Work out the finished part from the listing and answer in its coordinate system (mm). Give positions to 0.01 mm unless a question says otherwise; leave off trailing zeros. Loops run counter-clockwise (first coordinate to the right, second up) from the corner with the lowest first, then second, coordinate; pieces in that order, holes last. Notation, with made-up numbers: M -23,3 L 12,3 A23 ccw 12,29 Z; hole C -3.75,84 d10. An arc over 180 degrees is marked long. Answer in a Markdown table with one row per item. Add a question column.
from build123d import *

# Parameters (mm, degrees)
SKETCH1_R             = 92.075
BOSS_EXTRUDE1_DEPTH   = 4.7625
FILLET1_R             = 6.35
SKETCH4_R             = 1.5875
CUT_EXTRUDE1_DEPTH    = 131.30077765
SKETCH5_R             = 2.38125
CUT_EXTRUDE2_DEPTH    = 131.30077765
FRONTPATERNCOPY_COUNT = 18


with BuildPart() as part:
    # Sketch1 → Boss-Extrude1 (new body)
    with BuildSketch(Plane.XY):
        with Locations(Location((0, 0, 0), (0, 0, 180))):
            Circle(SKETCH1_R)
        with BuildLine():
            Line((-45.8597, 4.659861673), (-45.8597, 11.409392412))
            Line((-45.8597, 11.409392412), (-51.623596361, 20.547401417))
            ThreePointArc((-51.623596361, 20.547401417), (-49.007713262, 26.180822124), (-45.779418198, 31.487081093))
            Line((-45.779418198, 31.487081093), (-35.046071586, 32.720361416))
            Line((-35.046071586, 32.720361416), (-29.200806502, 36.095126785))
            ThreePointArc((-29.200806502, 36.095126785), (-27.113011458, 44.379898214), (-18.894291413, 42.045596046))
            Line((-18.894291413, 42.045596046), (-13.04902633, 45.420361416))
            Line((-13.04902633, 45.420361416), (-8.017226572, 54.981046592))
            ThreePointArc((-8.017226572, 54.981046592), (-1.830599579, 55.532335728), (4.378903018, 55.389679676))
            Line((4.378903018, 55.389679676), (10.813628414, 46.710969004))
            Line((10.813628414, 46.710969004), (16.658893498, 43.336203635))
            ThreePointArc((16.658893498, 43.336203635), (24.877613542, 45.670505803), (26.965408587, 37.385734374))
            Line((26.965408587, 37.385734374), (32.81067367, 34.010969004))
            Line((32.81067367, 34.010969004), (43.606369789, 34.433645175))
            ThreePointArc((43.606369789, 34.433645175), (47.177113682, 29.351513604), (50.158321216, 23.902598583))
            Line((50.158321216, 23.902598583), (45.8597, 13.990607588))
            Line((45.8597, 13.990607588), (45.8597, 7.241076849))
            ThreePointArc((45.8597, 7.241076849), (51.990625, 1.290607588), (45.8597, -4.659861673))
            Line((45.8597, -4.659861673), (45.8597, -11.409392412))
            Line((45.8597, -11.409392412), (51.623596361, -20.547401417))
            ThreePointArc((51.623596361, -20.547401417), (49.007713262, -26.180822124), (45.779418198, -31.487081093))
            Line((45.779418198, -31.487081093), (35.046071586, -32.720361416))
            Line((35.046071586, -32.720361416), (29.200806502, -36.095126785))
            ThreePointArc((29.200806502, -36.095126785), (27.113011458, -44.379898214), (18.894291413, -42.045596046))
            Line((18.894291413, -42.045596046), (13.04902633, -45.420361416))
            Line((13.04902633, -45.420361416), (8.017226572, -54.981046592))
            ThreePointArc((8.017226572, -54.981046592), (1.830599579, -55.532335728), (-4.378903018, -55.389679676))
            Line((-4.378903018, -55.389679676), (-10.813628414, -46.710969004))
            Line((-10.813628414, -46.710969004), (-16.658893498, -43.336203635))
            ThreePointArc((-16.658893498, -43.336203635), (-24.877613542, -45.670505803), (-26.965408587, -37.385734374))
            Line((-26.965408587, -37.385734374), (-32.81067367, -34.010969004))
            Line((-32.81067367, -34.010969004), (-43.606369789, -34.433645175))
            ThreePointArc((-43.606369789, -34.433645175), (-47.177113682, -29.351513604), (-50.158321216, -23.902598583))
            Line((-50.158321216, -23.902598583), (-45.8597, -13.990607588))
            Line((-45.8597, -13.990607588), (-45.8597, -7.241076849))
            ThreePointArc((-45.8597, -7.241076849), (-51.990625, -1.290607588), (-45.8597, 4.659861673))
        make_face(mode=Mode.SUBTRACT)
    extrude(amount=BOSS_EXTRUDE1_DEPTH)

    # Fillet1
    fillet1_edges = [part.edges().sort_by_distance(p)[0] for p in [
        (-43.606369789, -34.433645175, 2.38125),
        (-4.378903018, -55.389679676, 2.38125),
        (8.017226572, -54.981046592, 2.38125),
        (45.779418198, -31.487081093, 2.38125),
        (51.623596361, -20.547401417, 2.38125),
        (50.158321216, 23.902598583, 2.38125),
        (43.606369789, 34.433645175, 2.38125),
        (4.378903018, 55.389679676, 2.38125),
        (-8.017226572, 54.981046592, 2.38125),
        (-45.779418198, 31.487081093, 2.38125),
        (-51.623596361, 20.547401417, 2.38125),
        (-50.158321216, -23.902598583, 2.38125),
    ]]
    fillet(fillet1_edges, radius=FILLET1_R)

    # Sketch4 → Cut-Extrude1 (cut, through all)
    with BuildSketch(Plane.XY.offset(4.7625)):
        with Locations((-16.953011458, 50.011322779)):
            Circle(SKETCH4_R)
        with Locations((34.834570274, 39.687399983)):
            Circle(SKETCH4_R)
        with Locations((51.787581732, -10.323922796)):
            Circle(SKETCH4_R)
        with Locations((16.953011458, -50.011322779)):
            Circle(SKETCH4_R)
        with Locations((-34.834570274, -39.687399983)):
            Circle(SKETCH4_R)
        with Locations((-51.787581732, 10.323922796)):
            Circle(SKETCH4_R)
    extrude(amount=-CUT_EXTRUDE1_DEPTH, mode=Mode.SUBTRACT)

    # Sketch5 → Cut-Extrude2 (cut, through all)
    with BuildSketch(Plane.XY.offset(4.7625)):
        with Locations((0, 86.36)):
            Circle(SKETCH5_R)
        with Locations((0, 73.66)):
            Circle(SKETCH5_R)
        with Locations((14.114123881, 80.045174165)):
            Circle(SKETCH5_R)
    cut_extrude2 = extrude(amount=-CUT_EXTRUDE2_DEPTH, mode=Mode.SUBTRACT)

    # FrontPaternCopy: Cut-Extrude2 ×18 about axis
    frontpaterncopy_axis = Axis((0, 0, 0), (0, 0, 1))
    for i in range(1, FRONTPATERNCOPY_COUNT):
        add(cut_extrude2.rotate(frontpaterncopy_axis, i * 360 / FRONTPATERNCOPY_COUNT), mode=Mode.SUBTRACT)


solid = part.part
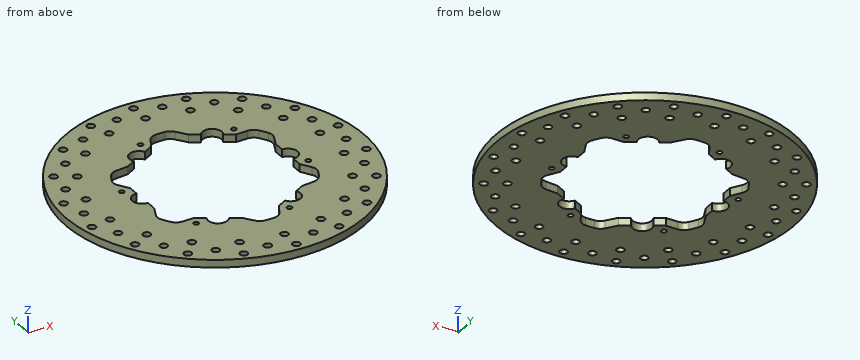
(1) Each of these flat-tipped pins is pushed along its axis until it touches: P1, Ø4.5, axis at x = 76.38, y = -27.8, coming from the +Z side; P2, Ø1.5, axis at x = -15, z = 2, coming from the +Y side; P3, Ø1.5, axis at x = -16.5, z = 2.5, coming from the -Y side. Where does it stop, or does it pass through?
(2) Consider line 1 along Y through (x, z) = (-2, 3.65); line 2 along Y through (x, z) = (-26, 2.45); line 3 along Y through (x, z) = (33.5, 1.35). Determine where each line is inside the solid, lowest interval first. Write a range as from..to.
(3) Section A-A, the plane y = -86.36 is taken. Determine the outline of the cut face in (x, z), and give its area (3 significant figures).
(4) Section B-B, the plane z = 3.05 is taken. State how many separate pieces and enclosed holes the cut face has, and give its area (3 significant figures).
Numbers:
| question | item | result |
|---|---|---|
| 1 | P1 | passes through |
| 1 | P2 | stops at y = 90.97 |
| 1 | P3 | stops at y = -90.72 |
| 2 | line 1 | y = -92.05..-87.65, -85.07..-74.95, -72.37..-55.48, 55.53..72.37, 74.95..85.07, 87.65..92.05 |
| 2 | line 2 | y = -88.33..-71.46, -66.98..-44.83, 44.88..66.98, 71.46..88.33 |
| 2 | line 3 | y = -85.76..-33.61, 34.04..38.83, 40.55..85.76 |
| 3 | outline | M -31.93,0 L -2.38,0 L -2.38,4.76 L -31.93,4.76 Z; M 2.38,0 L 31.93,0 L 31.93,4.76 L 2.38,4.76 Z |
| 3 | area | 281 mm² |
| 4 | separate pieces | 1 |
| 4 | enclosed holes | 61 |
| 4 | area | 17,500 mm² |
